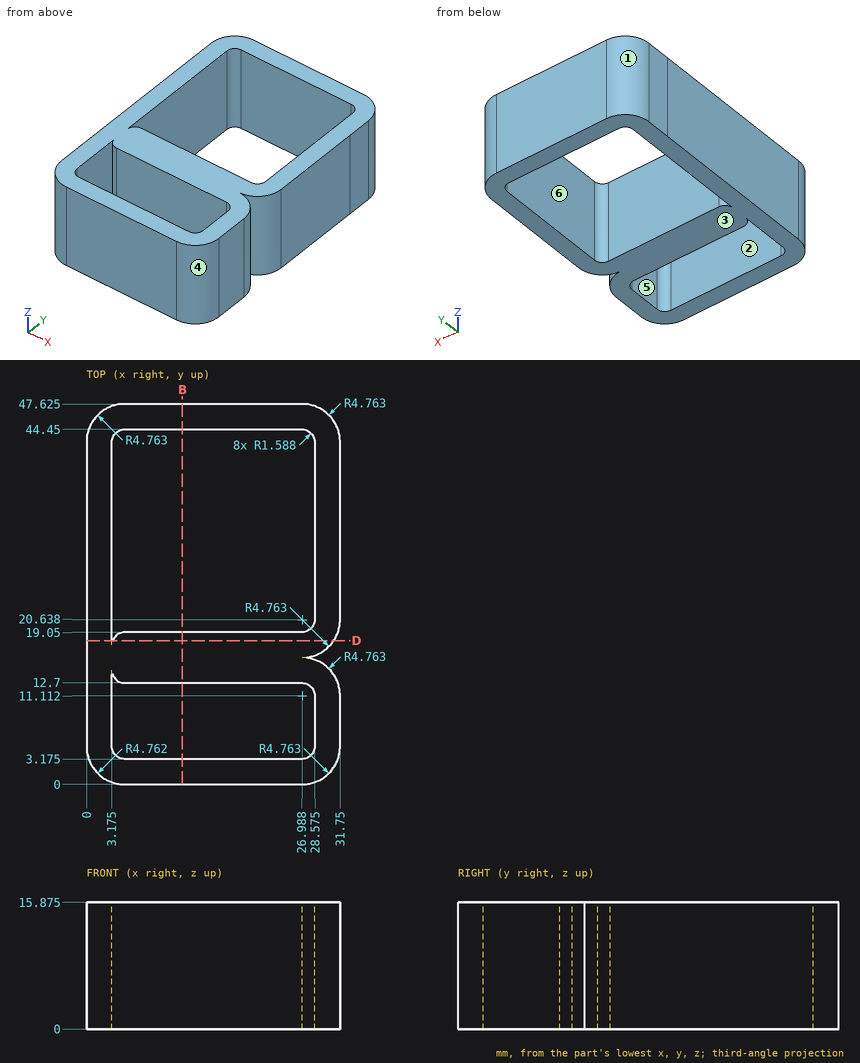
Geometry check sheet. Reference: drawing and pictorial views, mm from the part's lowest x, y, z. A direction names the side the tool comes from. Coordinates: 2 decimals unless noted, no trailing zeros. Loops run counter-clockwise (first coordinate to the right, second up) from the corner with the lowest first, then second, coordinate; pieces in that order, holes last. Notation, with made-up numbers: (-23.5, 17) -> (-0.5, 17) arc R21 cw to (-0.5, 23) -> close; hole circle Ø3 at (77, 1). An arc over 180 degrees is marked (long way). Write item = value, one per line. Start each with the question number.
1. Depth check by flat-ended pin: P1, Ø8, axis at x = 12.5, z = 8, coming from the -Y side; P2, Ø1, axis at x = 18, y = 11, coming from the +Z side. Enter the tip coordinate at first touch or a pass-through.
2. Section check D-D on y = 18. Record the cut outline in (x, z) (1 decimal), then the cut area to 3 significant figures.
3. Material ranges on line 1 (Y direction, x = 29, z = 14) (1 decimal); line 2 (Y direction, x = 3.5, z = 7.25) (1 decimal); line 3 (X direction, y = 43.5, z = 11.25), recorded low to high.
4. Tool access check on the marked faces 1 and 2. Record the directions out of +Z, -Z, +X, -X, +Y, -Y that give a thin tool (end or side, any length) a straight path to the whole face; none if there is none.
5. Section check B-B on x = 12. Give the number of separate pieces and of enclosed holes in the cut face.
6. Draft check along Y on the marked faces 3, 4, 5 and 6. Enter one of: released by +Y, released by -Y, zero draft, split by the parting line, or undercut.
Responses:
q1.P1 = 0
q1.P2 = through
q2.outline = (0, 0) -> (3.2, 0) -> (3.2, 15.9) -> (0, 15.9) -> close; (3.3, 0) -> (31, 0) -> (31, 15.9) -> (3.3, 15.9) -> close
q2.area = 490 mm2
q3.line_1 = 0.4 to 15.4, 16.3 to 47.2
q3.line_2 = 0.2 to 3.8, 13.3 to 18.4, 43.8 to 47.5
q3.line_3 = 0.04 to 3.31, 28.44 to 31.71
q4.face_1 = +Z, -Z, -X, +Y
q4.face_2 = +Z, -Z
q5.separate_pieces = 3
q5.enclosed_holes = 0
q6.face_3 = zero draft
q6.face_4 = released by -Y
q6.face_5 = undercut
q6.face_6 = undercut
